from build123d import *

# Parameters (mm, degrees)
SKETCH_6_W           = 42.3
SKETCH_6_H           = 42.3
SKETCH_6_R           = 1.6
SKETCH_6_R_2         = 15
EXTRUDE_1_DEPTH      = 5
SKETCH_7_R           = 1.6
SKETCH_7_R_2         = 4.15
EXTRUDE_5_DEPTH      = 38
EXTRUDE_START        = 38
SKETCH_7_7_R         = 4.15
SKETCH_7_7_R_2       = 1.6
EXTRUDE_7_DEPTH      = 38
SKETCH_7_8_R         = 4.15
SKETCH_7_8_R_2       = 1.6
EXTRUDE_8_DEPTH      = 38
SKETCH_12_W          = 2
SKETCH_12_H          = 44.3
EXTRUDE_11_DEPTH     = 38
SKETCH_14_W          = 44.3
SKETCH_14_H          = 2
EXTRUDE_12_DEPTH     = 38
SKETCH_15_W          = 2
SKETCH_15_H          = 42.3
EXTRUDE_13_DEPTH     = 38
CUT_EXTRUDE_1_DEPTH  = 13.2
CUT_EXTRUDE_2_DEPTH  = 123
SKETCH_19_R          = 1.5
CUT_EXTRUDE_3_DEPTH  = 10
EXTRUDE_15_DEPTH     = 11.2
EXTRUDE_16_DEPTH     = 11.2
EXTRUDE_17_DEPTH     = 2
SKETCH_26_R          = 1.6
SKETCH_26_R_2        = 15
CUT_EXTRUDE_10_DEPTH = 2
SKETCH_27_W          = 42.3
SKETCH_27_H          = 42.3
CUT_EXTRUDE_12_DEPTH = 5
SKETCH_29_W          = 46.3
SKETCH_29_H          = 38
EXTRUDE_18_DEPTH     = 2


with BuildPart() as part:
    # 草图6 → 凸台-拉伸1 (new body)
    with BuildSketch(Plane(origin=(0, 0, 0), x_dir=(1, 0, 0), z_dir=(0, 1, 0))):
        Rectangle(SKETCH_6_W, SKETCH_6_H)
        with Locations(Location((15.5, 15.5, 0), (0, 0, 270))):
            Circle(SKETCH_6_R, mode=Mode.SUBTRACT)
        with Locations(Location((-15.5, 15.5, 0), (0, 0, 270))):
            Circle(SKETCH_6_R, mode=Mode.SUBTRACT)
        with Locations(Location((-15.5, -15.5, 0), (0, 0, 270))):
            Circle(SKETCH_6_R, mode=Mode.SUBTRACT)
        with Locations(Location((15.5, -15.5, 0), (0, 0, 270))):
            Circle(SKETCH_6_R, mode=Mode.SUBTRACT)
        with Locations(Location((0, 0, 0), (0, 0, 270))):
            Circle(SKETCH_6_R_2, mode=Mode.SUBTRACT)
    extrude(amount=EXTRUDE_1_DEPTH)

    # 草图7 → 凸台-拉伸5 (add)
    # profile 1 of 2: a face of its own
    with BuildSketch(Plane(origin=(0, 5, 0), x_dir=(1, 0, 0), z_dir=(0, 1, 0))):
        with BuildLine():
            Line((49, -79), (49, -64))
            ThreePointArc((49, -64), (48.724429591, -61.789948347), (47.914593709, -59.715235547))
            Line((47.914593709, -59.715235547), (21.15, -10.277072187))
            Line((21.15, -10.277072187), (21.15, -21.15))
            Line((21.15, -21.15), (10.070005019, -21.15))
            Line((10.070005019, -21.15), (30.963898233, -65.919418373))
            Line((30.963898233, -65.919418373), (30.963898233, -79))
            Line((30.963898233, -79), (49, -79))
        make_face()
        with Locations(Location((40, -76, 0), (0, 0, 270))):
            Circle(SKETCH_7_R, mode=Mode.SUBTRACT)
        with Locations(Location((40, -64, 0), (0, 0, 270))):
            Circle(SKETCH_7_R_2, mode=Mode.SUBTRACT)
    # profile 2 of 2: a face of its own
    with BuildSketch(Plane(origin=(0, 5, 0), x_dir=(1, 0, 0), z_dir=(0, 1, 0))):
        with BuildLine():
            Line((-30.963898233, -65.919418373), (-10.070005019, -21.15))
            Line((-10.070005019, -21.15), (-21.15, -21.15))
            Line((-21.15, -21.15), (-21.15, -10.282583808))
            Line((-21.15, -10.282583808), (-46.202269248, -57.478354795))
            ThreePointArc((-46.202269248, -57.478354795), (-48.271046585, -60.45179082), (-49, -64))
            Line((-49, -64), (-49, -79))
            Line((-49, -79), (-30.963898233, -79))
            Line((-30.963898233, -79), (-30.963898233, -65.919418373))
        make_face()
        with Locations(Location((-40, -76, 0), (0, 0, 270))):
            Circle(SKETCH_7_R, mode=Mode.SUBTRACT)
        with Locations(Location((-40, -64, 0), (0, 0, 270))):
            Circle(SKETCH_7_R_2, mode=Mode.SUBTRACT)
    extrude(amount=-EXTRUDE_5_DEPTH)

    # 草图7<7> → 凸台-拉伸7 (add)
    with BuildSketch(Plane(origin=(0, 5, 0), x_dir=(1, 0, 0), z_dir=(0, 1, 0)).offset(EXTRUDE_START)):
        with Locations(Location((-40, -64, 0), (0, 0, 270))):
            Circle(SKETCH_7_7_R)
        with Locations(Location((40, -64, 0), (0, 0, 270))):
            Circle(SKETCH_7_7_R)
        with Locations(Location((40, -76, 0), (0, 0, 270))):
            Circle(SKETCH_7_7_R_2)
        with Locations(Location((-40, -76, 0), (0, 0, 270))):
            Circle(SKETCH_7_7_R_2)
    extrude(amount=-EXTRUDE_7_DEPTH)


with BuildPart() as extrude_7_kept_piece:
    # of the separate pieces the step leaves, the one the design keeps (extrude_7_pieces_kept)
    add(part.part.solids().sort_by_distance((-10.070005019, 0, 21.15))[0])

    # 草图7<8> → 凸台-拉伸8 (add)
    with BuildSketch(Plane(origin=(0, 5, 0), x_dir=(1, 0, 0), z_dir=(0, 1, 0))):
        with Locations(Location((-40, -64, 0), (0, 0, 270))):
            Circle(SKETCH_7_8_R)
        with Locations(Location((40, -64, 0), (0, 0, 270))):
            Circle(SKETCH_7_8_R)
        with Locations(Location((40, -76, 0), (0, 0, 270))):
            Circle(SKETCH_7_8_R_2)
        with Locations(Location((-40, -76, 0), (0, 0, 270))):
            Circle(SKETCH_7_8_R_2)
    extrude(amount=EXTRUDE_8_DEPTH)


with BuildPart() as extrude_8_kept_piece:
    # of the separate pieces the step leaves, the one the design keeps (extrude_8_pieces_kept)
    add(extrude_7_kept_piece.part.solids().sort_by_distance((-10.070005019, 0, 21.15))[0])

    # 草图12 → 凸台-拉伸11 (add)
    with BuildSketch(Plane(origin=(0, 5, 0), x_dir=(1, 0, 0), z_dir=(0, 1, 0))):
        with Locations((22.15, -1)):
            Rectangle(SKETCH_12_W, SKETCH_12_H)
    extrude(amount=-EXTRUDE_11_DEPTH)

    # 草图14 → 凸台-拉伸12 (add)
    with BuildSketch(Plane(origin=(0, 5, 0), x_dir=(1, 0, 0), z_dir=(0, 1, 0))):
        with Locations((-1, -22.15)):
            Rectangle(SKETCH_14_W, SKETCH_14_H)
    extrude(amount=-EXTRUDE_12_DEPTH)

    # 草图15 → 凸台-拉伸13 (add)
    with BuildSketch(Plane(origin=(0, 5, 0), x_dir=(1, 0, 0), z_dir=(0, 1, 0))):
        with Locations((-22.15, 0)):
            Rectangle(SKETCH_15_W, SKETCH_15_H)
    extrude(amount=-EXTRUDE_13_DEPTH)

    # 草图17 → 切除-拉伸1 (cut)
    with BuildSketch(Plane.XZ.offset(33)):
        Polygon((62.040525686, 30.953335803), (62.040525686, -32.044280047), (-61.83718559, -32.044280047), (-61.83718559, 30.953335803), (-61.83718559, 85.06296978), (-8.604799232, 85.06296978), (62.040525686, 85.06296978), align=None)
    extrude(amount=-CUT_EXTRUDE_1_DEPTH, mode=Mode.SUBTRACT)

    # 草图18 → 切除-拉伸2 (cut)
    with BuildSketch(Plane(origin=(49, 0, 0), x_dir=(0, 0, -1), z_dir=(1, 0, 0))):
        Polygon((-79, -4), (-69.450510985, -4), (-69.450510985, -12.643215043), (-69.450510985, -19.8), (-79, -19.8), (-79, -12.643215043), align=None)
    extrude(amount=-CUT_EXTRUDE_2_DEPTH, mode=Mode.SUBTRACT)

    # 草图19 → 切除-拉伸3 (cut)
    with BuildSketch(Plane(origin=(0, 0, 0), x_dir=(-1, 0, 0), z_dir=(0, -1, 0))):
        with Locations(Location((0, -17.95, 0), (0, 0, 90))):
            Circle(SKETCH_19_R)
        with Locations(Location((0, 17.95, 0), (0, 0, 90))):
            Circle(SKETCH_19_R)
    extrude(amount=-CUT_EXTRUDE_3_DEPTH, mode=Mode.SUBTRACT)

    # 草图23 → 凸台-拉伸15 (add)
    with BuildSketch(Plane(origin=(0, -19.8, 0), x_dir=(-1, 0, 0), z_dir=(0, -1, 0))):
        Polygon((-21.15, 21.15), (-23.15, 21.15), (-23.15, -13.971368009), (-23.15, -23.15), (-11.003405272, -23.15), (11.003405272, -23.15), (23.15, -23.15), (23.15, -14.050367917), (23.15, 21.15), (21.15, 21.15), (21.15, -21.15), (-21.15, -21.15), align=None)
    extrude(amount=EXTRUDE_15_DEPTH)

    # 草图24 → 凸台-拉伸16 (add)
    with BuildSketch(Plane(origin=(0, -19.8, 0), x_dir=(-1, 0, 0), z_dir=(0, -1, 0))):
        Polygon((23.15, -23.15), (27.980230087, -23.15), (23.15, -14.050367917), align=None)
        Polygon((-23.15, -23.15), (-28.119083383, -23.15), (-23.15, -13.971368009), align=None)
    extrude(amount=EXTRUDE_16_DEPTH)

    # 草图25 → 凸台-拉伸17 (add)
    with BuildSketch(Plane.XZ.offset(31)):
        Polygon((28.119083383, 23.15), (-27.980230087, 23.15), (-23.15, 14.050367917), (-23.15, -21.15), (23.15, -21.15), (23.15, 13.971368009), align=None)
    extrude(amount=EXTRUDE_17_DEPTH)

    # 草图26 → 切除-拉伸10 (cut)
    with BuildSketch(Plane.XZ.offset(33)):
        with Locations(Location((-15.5, 15.5, 0), (0, 0, 90))):
            Circle(SKETCH_26_R)
        with Locations(Location((15.5, 15.5, 0), (0, 0, 90))):
            Circle(SKETCH_26_R)
        with Locations(Location((15.5, -15.5, 0), (0, 0, 90))):
            Circle(SKETCH_26_R)
        with Locations(Location((-15.5, -15.5, 0), (0, 0, 90))):
            Circle(SKETCH_26_R)
        with Locations(Location((0, 0, 0), (0, 0, 90))):
            Circle(SKETCH_26_R_2)
    extrude(amount=-CUT_EXTRUDE_10_DEPTH, mode=Mode.SUBTRACT)

    # 草图27 → 切除-拉伸12 (cut)
    with BuildSketch(Plane.XZ):
        Rectangle(SKETCH_27_W, SKETCH_27_H)
    extrude(amount=-CUT_EXTRUDE_12_DEPTH, mode=Mode.SUBTRACT)

    # 草图29 → 凸台-拉伸18 (add)
    with BuildSketch(Plane(origin=(0, 0, -21.15), x_dir=(-1, 0, 0), z_dir=(0, 0, -1))):
        with Locations((0, -14)):
            Rectangle(SKETCH_29_W, SKETCH_29_H)
    extrude(amount=EXTRUDE_18_DEPTH)


solid = extrude_8_kept_piece.part
Source: CAD feature listing. Evaluate the final solid. Frame: model axes, mm. A direction names the side the tool comes from. Coordinates: 2 decimals unless noted, no trailing zeros. Write each loop counter-clockwise with the first axis right and the second up, starting at its lowest first coordinate (ties: lowest second). Pieces come first, ordered by that corner, then holes. Notation, with made-up numbers: M 81.5,21.25 L 94.5,21.25 A20 cw 94.5,57.25 Z; hole C 26.25,65.5 d6. An arc over 180 degrees is marked long. Use a Markdown table: item, result.
1) Section B-B, the plane y = -10. Output: boundary loops of the cut face in (x, z).
Conclusion:
| item | result |
|---|---|
| outline | M -49,64 A9 ccw -46.2,57.48 L -23.15,14.05 L -23.15,-23.15 L 23.15,-23.15 L 23.15,13.97 L 47.91,59.72 A9 ccw 49,64 L 49,69.45 L 30.96,69.45 L 30.96,65.92 L 11,23.15 L -11,23.15 L -30.96,65.92 L -30.96,69.45 L -49,69.45 Z; hole C -40,64 d8.3; hole M -21.15,-21.15 L 21.15,-21.15 L 21.15,21.15 L -21.15,21.15 Z; hole C 40,64 d8.3 |
2) First-contact query: pin 1 Ø21 at (x, z) = (5, -8) entering from +Y; pin 2 Ø5 at (y, z) = (-0.5, 43.5) entering from -X; pin 3 Ø17.5 at (x, y) = (43, -11) entering from +Z; pin 4 Ø1 at (y, z) = (-20.5, 31) entering from -X. Flat tips, straight axial feed; report the tip coordinate or a pass-through.
Conclusion:
| item | result |
|---|---|
| pin 1 | stops at y = -31 |
| pin 2 | stops at x = -40.11 |
| pin 3 | stops at z = 79 |
| pin 4 | passes through |
3) Section C-C, the plane x = 0. Output: boundary loops of the cut face in (y, z).
Conclusion:
| item | result |
|---|---|
| outline | M -33,-23.15 L 5,-23.15 L 5,-21.15 L -31,-21.15 L -31,-15 L -33,-15 Z; M -33,15 L -31,15 L -31,21.15 L 5,21.15 L 5,23.15 L -33,23.15 Z |
4) Section D-D, the plane y = -29. Output: boundary loops of the cut face in (x, z), then the cut area to 3 significant figures.
Conclusion:
| item | result |
|---|---|
| outline | M -27.98,23.15 L -23.15,14.05 L -23.15,-23.15 L 23.15,-23.15 L 23.15,13.97 L 28.12,23.15 Z; hole M -21.15,-21.15 L 21.15,-21.15 L 21.15,21.15 L -21.15,21.15 Z |
| area | 399 mm^2 |
5) Ray query, L1, parallel to Z at x = 15.5, y = -32.4; L2, parallel to X at y = -1.5, z = 12. Return the intervals inside material, ascending.
Conclusion:
| item | result |
|---|---|
| L1 | z = -23.15 to -17.1, -13.9 to 13.9, 17.1 to 23.15 |
| L2 | x = -23.15 to -21.15, 21.15 to 23.15 |
6) Section A-A, the plane z = 0. Output: boundary loops of the cut face in (x, y), then the cut area to 3 significant figures.
Conclusion:
| item | result |
|---|---|
| outline | M -23.15,-33 L -15,-33 L -15,-31 L -21.15,-31 L -21.15,5 L -23.15,5 Z; M 15,-33 L 23.15,-33 L 23.15,5 L 21.15,5 L 21.15,-31 L 15,-31 Z |
| area | 177 mm^2 |
7) Reachability of faces 5 (the flat face through (0, -13, -21.15)), 6 (the flat face through (40, -4, 74)), 7 (the flat face through (20.844, -7.226, 44.235)), 8 (the flat face through (23.15, -14, -4)) from +Z, -Z, +X, -X, +Y, -Y: full face, straight path, thin tool, end or side. Return the list, or none.
Conclusion:
| item | result |
|---|---|
| face 5 | +Y |
| face 6 | +Z, +X, -X, -Y |
| face 7 | +Z, +Y, -Y |
| face 8 | -Z, +X, +Y, -Y |
8) Mould query, pull axis X, two halves, no side actions, for faces 1 (the flat face through (30.964, -2, 71)), 2 (the flat face through (-34.84, -9.51, 36.07)), 3 (the flat face through (49, -4, 68)), 4 (the cylindrical face through (-16.58, -32.01, 14.32)). Classes: pulls with the +X half, pulls with the -X half, needs draft (parallel to the pull), parting line crosses it, or undercut.
Conclusion:
| item | result |
|---|---|
| face 1 | undercut |
| face 2 | pulls with the -X half |
| face 3 | pulls with the +X half |
| face 4 | undercut |
